from build123d import *

# Parameters (mm, degrees)
SKETCH1_W           = 80
SKETCH1_H           = 60
BOSS_EXTRUDE5_DEPTH = 5
SKETCH4_W           = 80
SKETCH4_H           = 60
SKETCH4_W_2         = 75
SKETCH4_H_2         = 55
BOSS_EXTRUDE6_DEPTH = 30
FILLET2_R           = 5


with BuildPart() as part:
    # Sketch1 → Boss-Extrude5 (new body)
    with BuildSketch(Plane.XY):
        Rectangle(SKETCH1_W, SKETCH1_H)
    extrude(amount=-BOSS_EXTRUDE5_DEPTH)

    # Sketch4 → Boss-Extrude6 (add)
    with BuildSketch(Plane(origin=(0, 0, -5), x_dir=(-1, 0, 0), z_dir=(0, 0, -1))):
        Rectangle(SKETCH4_W, SKETCH4_H)
        Rectangle(SKETCH4_W_2, SKETCH4_H_2, mode=Mode.SUBTRACT)
    extrude(amount=BOSS_EXTRUDE6_DEPTH)

    # Fillet2
    fillet2_edges = [part.edges().sort_by_distance(p)[0] for p in [
        (40, -30, -17.5),
        (-40, -30, -17.5),
        (-40, 30, -17.5),
        (40, 30, -17.5),
    ]]
    fillet(fillet2_edges, radius=FILLET2_R)


solid = part.part
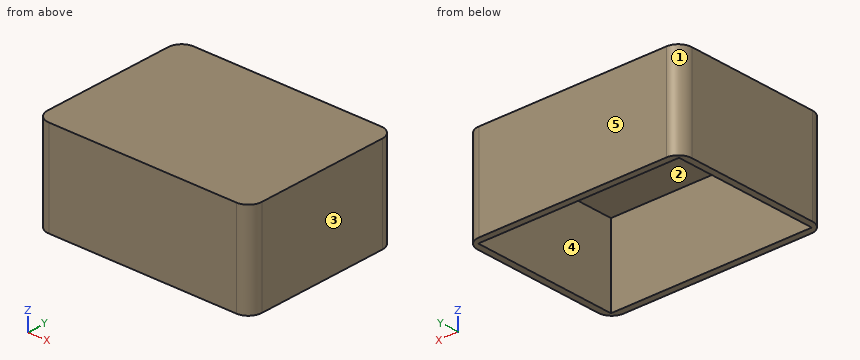
Geometry check sheet. Reference: the model listing, model coordinates, mm. Face numbers are marked on the shaded views. A direction names the side the tool comes from. Coordinates: 2 decimals unless noted, no trailing zeros. Loops run counter-clockwise (first coordinate to the right, second up) from the corner with the lowest first, then second, coordinate; pieces in that order, holes last. Notation, with made-up numbers: (52, 8.5) - (60, 8.5) arc R33 ccw to (60, 45.5) - close; hole circle Ø1 at (57.25, 50). An arc over 180 degrees is marked (long way). Use one line per item in the form item = value. Start each with the question number.
Item 1: Mould release check, pull along X, two halves, no side actions. Record for the marked faces 3, 4 and 5: +X half, -X half, draft (parallel to the pull), parting line (faces both ways), or undercut.
Item 2: Gauge pin test, flat end, axial feed: pin 1 (16.5 mm diameter, centred on x = 2.5, y = -13, fed in from -Z). Record the tip position at first contact, or that the pin passes through.
Item 3: Section check C-C, the plane y = 21.5. Enter the section's corners in (x, z), and give its area (3 significant figures).
Item 4: Section check B-B, the plane x = 31. Enter the section's corners in (y, z).
Item 5: Tool access check on the marked faces 1 and 2. Record the directions out of +Z, -Z, +X, -X, +Y, -Y that give a thin tool (end or side, any length) a straight path to the whole face; none if there is none.
Item 6: Section check A-A, the plane z = -7.5. Enter the section's corners in (x, y), and give its area (3 significant figures).
Item 7: Thickness scan on probe 1 along X at (y, z) = (9, -25.5); probe 2 along Y at (x, z) = (-4.5, -21); probe 3 along Z at (x, y) = (16, -6). Record the ranges inside material, lowest first.
Computed:
q1.face_3 = +X half
q1.face_4 = undercut
q1.face_5 = draft
q2.pin_1 = -5
q3.outline = (-40, -35) - (-37.5, -35) - (-37.5, -5) - (37.5, -5) - (37.5, -35) - (40, -35) - (40, 0) - (-40, 0) - close
q3.area = 550 mm2
q4.outline = (-30, -35) - (-27.5, -35) - (-27.5, -5) - (27.5, -5) - (27.5, -35) - (30, -35) - (30, 0) - (-30, 0) - close
q5.face_1 = +Z, -Z, -X, +Y
q5.face_2 = -Z
q6.outline = (-40, -25) arc R5 ccw to (-35, -30) - (35, -30) arc R5 ccw to (40, -25) - (40, 25) arc R5 ccw to (35, 30) - (-35, 30) arc R5 ccw to (-40, 25) - close; hole (-37.5, -27.5) - (37.5, -27.5) - (37.5, 27.5) - (-37.5, 27.5) - close
q6.area = 654 mm2
q7.probe_1 = -40 to -37.5, 37.5 to 40
q7.probe_2 = -30 to -27.5, 27.5 to 30
q7.probe_3 = -5 to 0
